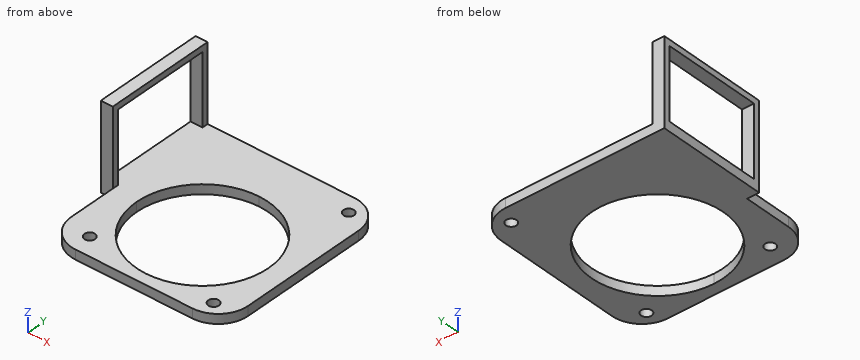
from build123d import *

# Parameters (mm, degrees)
F1_R     = 2.25
F2_DEPTH = 4
F3_W     = 46.78
F3_H     = 4
F3_H_2   = 32.54
F4_DEPTH = 5.08
F5_W     = 41.7
F5_H     = 30
F6_DEPTH = 25.4


with BuildPart() as f2:
    # F1 (on Top) → F2 (new body)
    with BuildSketch(Plane.XY):
        with BuildLine():
            Line((6.9206423996, 43.995959647), (-16.8793576004, 43.995959647))
            Line((-16.8793576004, 43.995959647), (-16.8793576004, 24.595959647))
            ThreePointArc((-16.8793576004, 24.595959647), (2.8772058659, 16.4125231134), (11.0606423996, -3.344040353))
            Line((11.0606423996, -3.344040353), (19.6206423996, -3.344040353))
            Line((19.6206423996, -3.344040353), (19.6206423996, 31.295959647))
            ThreePointArc((19.6206423996, 31.295959647), (15.9008985206, 40.2762157681), (6.9206423996, 43.995959647))
        make_face()
        with Locations((10.7806423996, 36.655959647)):
            Circle(F1_R, mode=Mode.SUBTRACT)
        with BuildLine():
            Line((19.6206423996, -3.344040353), (11.0606423996, -3.344040353))
            ThreePointArc((11.0606423996, -3.344040353), (2.8772058659, -23.1006038194), (-16.8793576004, -31.284040353))
            Line((-16.8793576004, -31.284040353), (-16.8793576004, -36.004040353))
            Line((-16.8793576004, -36.004040353), (6.9206423996, -36.004040353))
            ThreePointArc((6.9206423996, -36.004040353), (15.9008985206, -32.2842964741), (19.6206423996, -23.304040353))
            Line((19.6206423996, -23.304040353), (19.6206423996, -3.344040353))
        make_face()
        with Locations((10.1206423996, -29.264040353)):
            Circle(F1_R, mode=Mode.SUBTRACT)
        with BuildLine():
            Line((-44.8193576004, -3.344040353), (-55.3793576004, -3.344040353))
            Line((-55.3793576004, -3.344040353), (-55.3793576004, -23.304040353))
            ThreePointArc((-55.3793576004, -23.304040353), (-51.6596137215, -32.2842964741), (-42.6793576004, -36.004040353))
            Line((-42.6793576004, -36.004040353), (-16.8793576004, -36.004040353))
            Line((-16.8793576004, -36.004040353), (-16.8793576004, -31.284040353))
            ThreePointArc((-16.8793576004, -31.284040353), (-36.6359210668, -23.1006038194), (-44.8193576004, -3.344040353))
        make_face()
        with Locations((-43.8793576004, -27.554040353)):
            Circle(F1_R, mode=Mode.SUBTRACT)
        with BuildLine():
            Line((-16.8793576004, 43.995959647), (-55.3793576004, 43.995959647))
            Line((-55.3793576004, 43.995959647), (-55.3793576004, -3.344040353))
            Line((-55.3793576004, -3.344040353), (-44.8193576004, -3.344040353))
            ThreePointArc((-44.8193576004, -3.344040353), (-36.6359210668, 16.4125231134), (-16.8793576004, 24.595959647))
            Line((-16.8793576004, 24.595959647), (-16.8793576004, 43.995959647))
        make_face()
    extrude(amount=F2_DEPTH)

    # F3 (on face) → F4 (join)
    with BuildSketch(Plane(origin=(-55.3793576004, 0, 0), x_dir=(0, -1, 0), z_dir=(-1, 0, 0))):
        with Locations((-20.605959647, 2)):
            Rectangle(F3_W, F3_H)
        with Locations((-20.605959647, 20.27)):
            Rectangle(F3_W, F3_H_2)
    extrude(amount=F4_DEPTH)

    # F5 (on face) → F6 (cut)
    with BuildSketch(Plane(origin=(-60.4593576004, 0, 0), x_dir=(0, -1, 0), z_dir=(-1, 0, 0))):
        with Locations((-20.605959647, 19)):
            Rectangle(F5_W, F5_H)
    extrude(amount=-F6_DEPTH, mode=Mode.SUBTRACT)


solid = f2.part
Source: CAD feature listing. Evaluate the final solid. Frame: model axes, mm. Give positions to 0.01 mm unless a question says otherwise; leave off trailing zeros. Write each loop counter-clockwise with the first axis right and the second up, starting at its lowest first coordinate (ties: lowest second). Pieces come first, ordered by that corner, then holes. Notation, with made-up numbers: M 18.5,48.5 L 32.5,48.5 A7 ccw 32.5,58.5 Z; hole C 11.5,75 d6. An arc over 180 degrees is marked long. Return JSON: item names as keys, results as strings. Group by question number.
1) Cut plane A-A, the plane y = 29. Output: boundary loops of the cut face in (x, z), plus the area to 3 significant figures.
2) Pin query (flat end, axial travel): P1, Ø6, axis at y = 14, z = 6, coming from the +X side; P2, Ø1.5, axis at x = -59, z = 11.5, coming from the -Y side; P3, Ø4.5, axis at y = -8.5, z = 3, coming from the -X side; P4, Ø7, axis at x = 10.78, y = 36.66, coming from the +Z side. Return the tip coordinate at first contact, or that it passes through.
3) Cut plane C-C, the plane y = 7. Output: boundary loops of the cut face in (x, z), plus the area to 3 significant figures.
4) Material intervals for line 1 along Z through (x, y) = (-10.5, 33); line 2 along Y through (x, z) = (4.5, 3.5); line 3 along X through (y, z) = (-6.5, 3.5), sorted ascending. Write a range as [from, to].
5) Cut plane B-B, the plane z = 16.5. Output: boundary loops of the cut face in (x, y).
6) Cut plane D-D, the plane z = 2. Output: boundary loops of the cut face in (x, y).
Recorded:
{
 "1": {"outline": "M -60.46,0 L 19.62,0 L 19.62,4 L -60.46,4 Z; M -60.46,34 L -55.38,34 L -55.38,36.54 L -60.46,36.54 Z", "area": "333 mm²"},
 "2": {"P1": "stops at x = 19.62", "P2": "stops at y = -2.78", "P3": "stops at x = -55.38", "P4": "stops at z = 4"},
 "3": {"outline": "M -60.46,0 L -42.83,0 L -42.83,4 L -60.46,4 Z; M -60.46,34 L -55.38,34 L -55.38,36.54 L -60.46,36.54 Z; M 9.08,0 L 19.62,0 L 19.62,4 L 9.08,4 Z", "area": "126 mm²"},
 "4": {"line 1": "z = [0, 4]", "line 2": "y = [-36, -21.33], [14.64, 44]", "line 3": "x = [-55.38, -44.64], [10.88, 19.62]"},
 "5": {"outline": "M -60.46,-2.78 L -55.38,-2.78 L -55.38,-0.24 L -60.46,-0.24 Z; M -60.46,41.46 L -55.38,41.46 L -55.38,44 L -60.46,44 Z"},
 "6": {"outline": "M -60.46,-2.78 L -55.38,-2.78 L -55.38,-23.3 A12.7 ccw -42.68,-36 L 6.92,-36 A12.7 ccw 19.62,-23.3 L 19.62,31.3 A12.7 ccw 6.92,44 L -60.46,44 Z; hole C -43.88,-27.55 d4.5; hole C -16.88,-3.34 d55.88; hole C 10.12,-29.26 d4.5; hole C 10.78,36.66 d4.5"}
}
